The listing builds one solid part. Answer for the finished solid, in the listing's coordinates (mm). A direction names the side the tool comes from. Coordinates: 2 decimals unless noted, no trailing zeros. Loops run counter-clockwise (first coordinate to the right, second up) from the corner with the lowest first, then second, coordinate; pieces in that order, holes last. Notation, with made-up numbers: (-38, -35) - (-7, -35) arc R25 cw to (-7, -14) - close; hole circle Ø4 at (9, 65). An arc over 180 degrees is marked (long way). Put each result on its own line as item: value.
```python
from build123d import *

# Parameters (mm, degrees)
SKETCH1_W           = 34.798
SKETCH1_H           = 41.656
BOSS_EXTRUDE2_DEPTH = 111.506
SKETCH2_W           = 30.48
SKETCH2_H           = 38.1
BOSS_EXTRUDE3_DEPTH = 29.464
SKETCH3_R           = 6.35
CUT_EXTRUDE2_DEPTH  = 12.7
SKETCH4_R           = 6.35
CUT_EXTRUDE3_DEPTH  = 12.7


with BuildPart() as part:
    # Sketch1 → Boss-Extrude2 (new body)
    with BuildSketch(Plane.XY):
        with Locations((17.399, 20.828)):
            Rectangle(SKETCH1_W, SKETCH1_H)
    extrude(amount=BOSS_EXTRUDE2_DEPTH)

    # Sketch2 → Boss-Extrude3 (add)
    with BuildSketch(Plane.XY.offset(111.506)):
        with Locations((16.764, 19.05)):
            Rectangle(SKETCH2_W, SKETCH2_H)
    boss_extrude3 = extrude(amount=BOSS_EXTRUDE3_DEPTH)

    # Mirror1: Boss-Extrude3 across plane
    add(boss_extrude3.mirror(Plane(origin=(0, 0, 55.753), x_dir=(1, 0, 0), z_dir=(0, 0, -1))))

    # Sketch3 → Cut-Extrude2 (cut)
    with BuildSketch(Plane.XZ):
        with Locations((16.764, 55.753)):
            Circle(SKETCH3_R)
    extrude(amount=-CUT_EXTRUDE2_DEPTH, mode=Mode.SUBTRACT)

    # Sketch4 → Cut-Extrude3 (cut)
    with BuildSketch(Plane(origin=(0, 41.656, 0), x_dir=(1, 0, 0), z_dir=(0, 1, 0))):
        with Locations((17.399, -43.053)):
            Circle(SKETCH4_R)
        with Locations((17.399, -68.453)):
            Circle(SKETCH4_R)
    extrude(amount=-CUT_EXTRUDE3_DEPTH, mode=Mode.SUBTRACT)


solid = part.part
```
1) The part is cut by section B-B (y = 18.5). Give the vertices of the cut face in (x, z), and give its area (3 significant figures).
Found:
outline: (0, 0) - (1.52, 0) - (1.52, -29.46) - (32, -29.46) - (32, 0) - (34.8, 0) - (34.8, 111.51) - (32, 111.51) - (32, 140.97) - (1.52, 140.97) - (1.52, 111.51) - (0, 111.51) - close
area: 5,680 mm^2
2) The part is cut by section A-A (x = 30). Give the vertices of the cut face in (y, z), and give its area (3 significant figures).
Found:
outline: (0, -29.46) - (38.1, -29.46) - (38.1, 0) - (41.66, 0) - (41.66, 111.51) - (38.1, 111.51) - (38.1, 140.97) - (0, 140.97) - close
area: 6,890 mm^2
3) Each of these flat-tipped pins is pushed along its axis until it touches: pin 1 (5 mm diameter, centred on x = 11, z = 117, fed in from +Y); pin 2 (4 mm diameter, centred on x = 16, z = 55, fed in from -Y); pin 3 (4 mm diameter, centred on y = 19, z = -7.5, fed in from -X). Where does it stop, or does it pass through?
Found:
pin 1: stops at y = 38.1
pin 2: stops at y = 12.7
pin 3: stops at x = 1.52
4) For faces 1 (the face through (16.02, 35.39, 49.25)), 2 (the face through (15.387, 6.261, 49.554)), 3 (the face through (32.004, 19, -15)), 4 (the face through (17, 38.1, -15)), determine the directions among +Z, -Z, +X, -X, +Y, -Y from which every point of the face is accessible in a straight line to the end or side of a thin tool.
Found:
face 1: +Y
face 2: -Y
face 3: -Z, +X, +Y, -Y
face 4: -Z, +X, -X, +Y
5) The part is cut by section D-D (y = 8). Give the vertices of the cut face in (x, z), and give its area (3 significant figures).
Found:
outline: (0, 0) - (1.52, 0) - (1.52, -29.46) - (32, -29.46) - (32, 0) - (34.8, 0) - (34.8, 111.51) - (32, 111.51) - (32, 140.97) - (1.52, 140.97) - (1.52, 111.51) - (0, 111.51) - close; hole circle Ø12.7 at (16.76, 55.75)
area: 5,550 mm^2
6) For a pull along X with two mould halves and no side action, classify faces 5 (the face through (17, 19, 140.97)), 6 (the face through (16.02, 35.39, 74.65)), 7 (the face through (17, 28.956, 43)), 8 (the face through (1.524, 19, 126)) as pulls with the +X half, pulls with the -X half, needs draft (parallel to the pull), parting line crosses it, or undercut.
Found:
face 5: needs draft
face 6: undercut
face 7: undercut
face 8: pulls with the -X half
7) The part is cut by section C-C (z = 52). Give the vertices of the cut face in (x, y).
Found:
outline: (0, 0) - (11.64, 0) - (11.64, 12.7) - (21.89, 12.7) - (21.89, 0) - (34.8, 0) - (34.8, 41.66) - (0, 41.66) - close
8) Straight lines are drawn through the part: L1, parallel to Y at x = 11.5, z = 69; L2, parallel to Y at x = 17.5, z = 49.5; L3, parallel to X at y = 11, z = -17. For each, find the intervals that lie inside material, in ascending order. Write a range as [from, to].
Found:
L1: y = [0, 28.96]
L2: y = [12.7, 41.66]
L3: x = [1.52, 32]
